```python
from build123d import *
from build123d.topology import SkipClean

# Parameters (mm, degrees)
SKETCH2_R                      = 31.5
BOSS_EXTRUDE1_DEPTH            = 12
CBORE_FOR_M6_SHCS1_D           = 6.4
CBORE_FOR_M6_SHCS1_CBORE_D     = 11
CBORE_FOR_M6_SHCS1_CBORE_DEPTH = 6.5
SKETCH5_R                      = 3.15
CUT_EXTRUDE1_DEPTH             = 12
BOSS_EXTRUDE2_DEPTH            = 24.5
CUT_EXTRUDE2_START             = 65
SKETCH7_R                      = 5.5
CUT_EXTRUDE2_DEPTH             = 65
BOSS_EXTRUDE3_REACH            = 66.882
CUT_EXTRUDE3_START             = 82
SKETCH9_R                      = 5.5
CUT_EXTRUDE3_DEPTH             = 82
SKETCH11_R                     = 51.4472096
SKETCH11_R_2                   = 31.5
CUT_EXTRUDE4_DEPTH             = 82
SKETCH12_R                     = 1.6
CUT_EXTRUDE5_DEPTH             = 52


with BuildPart() as part:
    # Sketch2 → Boss-Extrude1 (new body)
    with BuildSketch(Plane.XY):
        Circle(SKETCH2_R)
    extrude(amount=BOSS_EXTRUDE1_DEPTH)

    # CBORE for M6 SHCS1 (through all)
    with Locations(Plane.XY.offset(12)):
        with Locations((0, 25), (0, -25)):
            CounterBoreHole(CBORE_FOR_M6_SHCS1_D / 2, CBORE_FOR_M6_SHCS1_CBORE_D / 2, CBORE_FOR_M6_SHCS1_CBORE_DEPTH)

    # Sketch5 → Cut-Extrude1 (cut)
    with BuildSketch(Plane(origin=(0, 0, 0), x_dir=(-1, 0, 0), z_dir=(0, 0, -1))):
        with Locations((17.67766953, 17.67766953)):
            Circle(SKETCH5_R)
    extrude(amount=-CUT_EXTRUDE1_DEPTH, mode=Mode.SUBTRACT)

    # Sketch6 → Boss-Extrude2 (add)
    with BuildSketch(Plane(origin=(17.25, 0, 0), x_dir=(0, 0, -1), z_dir=(1, 0, 0))):
        Polygon((-12, 29.231895539), (-28.9984059, 19.417861316), (-12, -10.02424135), align=None)
    extrude(amount=-BOSS_EXTRUDE2_DEPTH)

    # Sketch7 → Cut-Extrude2 (cut)
    with BuildSketch(Plane.XY.offset(12).offset(CUT_EXTRUDE2_START)):
        with Locations((0, 25)):
            Circle(SKETCH7_R)
    extrude(amount=-CUT_EXTRUDE2_DEPTH, mode=Mode.SUBTRACT)

    # Boss-Extrude3: up to this face of the body (flat: up to its plane)
    boss_extrude3_end = Plane(part.part.faces().sort_by_distance((-7.25, 12.875171835, 17.6661353))[0])
    # Sketch8 → Boss-Extrude3 (add, up to the picked face)
    with BuildSketch(Plane(origin=(17.25, 0, 0), x_dir=(0, 0, -1), z_dir=(1, 0, 0)), mode=Mode.PRIVATE) as boss_extrude3_sk1:
        Polygon((-12, -10.02424135), (-20.878095029, -15.150011905), (-12, -30.52732357), align=None)
    boss_extrude3_tool1 = split(extrude(boss_extrude3_sk1.sketch, amount=-BOSS_EXTRUDE3_REACH, mode=Mode.PRIVATE), bisect_by=boss_extrude3_end, keep=Keep.BOTH, mode=Mode.PRIVATE)
    add(boss_extrude3_tool1.solids().sort_by(Axis((17.25, -18.567192, 14.959365), (-1, 0, 0)))[0])

    # Sketch9 → Cut-Extrude3 (cut)
    with BuildSketch(Plane.XY.offset(12).offset(CUT_EXTRUDE3_START)):
        with Locations((0, -25)):
            Circle(SKETCH9_R)
    extrude(amount=-CUT_EXTRUDE3_DEPTH, mode=Mode.SUBTRACT)

    # Sketch11 → Cut-Extrude4 (cut)
    with SkipClean():  # the faces are left unmerged after this step: merging them gives an invalid solid
        with BuildSketch(Plane(origin=(0, 0, 0), x_dir=(-1, 0, 0), z_dir=(0, 0, -1))):
            Circle(SKETCH11_R)
            with Locations(Location((0, 0, 0), (0, 0, 255.72452839))):
                Circle(SKETCH11_R_2, mode=Mode.SUBTRACT)
        extrude(amount=-CUT_EXTRUDE4_DEPTH, mode=Mode.SUBTRACT)
    add(part.part.scale(1), mode=Mode.REPLACE)  # the faces are merged on a copy

    # Sketch12 → Cut-Extrude5 (cut)
    with BuildSketch(Plane.ZY.offset(7.25)):
        with Locations((19.788303121, 18.963925862)):
            Circle(SKETCH12_R)
        with Locations((15.278684177, -18.84696327)):
            Circle(SKETCH12_R)
    extrude(amount=-CUT_EXTRUDE5_DEPTH, mode=Mode.SUBTRACT)


solid = part.part
```
Source: CAD feature listing. Evaluate the final solid. Frame: model axes, mm. A direction names the side the tool comes from. Give positions to 0.01 mm unless a question says otherwise; leave off trailing zeros. Loops run counter-clockwise (first coordinate to the right, second up) from the corner with the lowest first, then second, coordinate; pieces in that order, holes last. Notation, with made-up numbers: (13.5, 43.25) -> (31.5, 43.25) arc R21 ccw to (31.5, 72.25) -> close; hole circle Ø2 at (-40, 57.5). An arc over 180 degrees is marked (long way). Use a Markdown table: item, result. Add a question column.
(1) Section query C-C (x = 0). Count the separate pieces of the cut face and the enclosed holes in it, then the cut area to 3 significant figures.
(2) Ray query, line 1 (Y direction, x = 0, z = 11.75); line 2 (Y direction, x = 0, z = 2.45); line 3 (Z direction, x = -10, y = 27). Return the intervals inside material, ascending.
(3) Section query A-A (x = -20). Output: boundary loops of the cut face in (y, z), then the cut area to 3 significant figures.
(4) Section query D-D (y = 8.5). Output: boundary loops of the cut face in (x, z), then the cut area to 3 significant figures.
(5) First-contact query: pin 1 Ø5 at (y, z) = (-18.85, 15.28) entering from -X; pin 2 Ø2.5 at (y, z) = (-22, 16.5) entering from +X; pin 3 Ø1 at (y, z) = (-19.5, 15) entering from +X; pin 4 Ø10 at (x, y) = (0, -25) entering from -Z. Flat tips, straight axial feed; report the tip coordinate or a pass-through.
(6) Access query for faces 1 (the face through (5.172, 4.903, 20.618)), 2 (the face through (-7.25, 14, 17)), 3 (the face through (-1.19, 19.63, 14.78)). Directions: +Z, -Z, +X, -X, +Y, -Y. A direction counts if a zero-diameter tool reaches every point of the face in a straight line with its end or side. Return the directions, or none.
(7) Section query B-B (y = -23). Output: boundary loops of the cut face in (x, z).
(8) Pull-direction query (X, two-part tool) for faces 4 (the face through (7.894, 24.394, 20.38)), 5 (the face through (0.417, 28.173, 2.712)), 6 (the face through (2.4, 22.6, 5.5)), 7 (the face through (17.25, 12, 19)); classes: +X half, -X half, draft (parallel to the pull), parting line (faces both ways), or undercut.
Checked values:
| question | item | result |
|---|---|---|
| 1 | separate pieces | 3 |
| 1 | enclosed holes | 0 |
| 1 | area | 838 mm^2 |
| 2 | line 1 | -31.5 to -30.5, -19.5 to 19.5, 30.5 to 31.5 |
| 2 | line 2 | -31.5 to -28.2, -21.8 to 21.8, 28.2 to 31.5 |
| 2 | line 3 | 0 to 12 |
| 3 | outline | (-24.34, 0) -> (15.55, 0) -> (15.55, 12) -> (-24.34, 12) -> close; (19.81, 0) -> (24.34, 0) -> (24.34, 12) -> (19.81, 12) -> close |
| 3 | area | 533 mm^2 |
| 4 | outline | (-30.33, 0) -> (30.33, 0) -> (30.33, 12) -> (17.25, 12) -> (17.25, 22.69) -> (-7.25, 22.69) -> (-7.25, 12) -> (-30.33, 12) -> close |
| 4 | area | 990 mm^2 |
| 5 | pin 1 | x = -7.25 |
| 5 | pin 2 | x = 17.25 |
| 5 | pin 3 | through |
| 5 | pin 4 | z = 0 |
| 6 | face 1 | +Z, +X, -X |
| 6 | face 2 | +Z, -X, +Y, -Y |
| 6 | face 3 | +Z |
| 7 | outline | (-21.52, 0) -> (-2.5, 0) -> (-2.5, 5.5) -> (-5.12, 5.5) -> (-5.12, 16.35) -> (-7.25, 16.35) -> (-7.25, 12) -> (-21.52, 12) -> close; (2.5, 0) -> (21.52, 0) -> (21.52, 12) -> (17.25, 12) -> (17.25, 16.35) -> (5.12, 16.35) -> (5.12, 5.5) -> (2.5, 5.5) -> close |
| 8 | face 4 | draft |
| 8 | face 5 | undercut |
| 8 | face 6 | undercut |
| 8 | face 7 | +X half |
